Geometry check sheet. Reference: the model listing, model coordinates, mm. A direction names the side the tool comes from. Round coordinates to 2 decimals unless told otherwise and drop trailing zeros. Order: outer loops, then holes, each group sorted by start corner. A loop starts at its lowest first (then second) coordinate and runs counter-clockwise, first axis right, second up.
(1) Sectioned sample at D-D (z = 25.5). Record the boundary of the cut face in (x, y), plus the area to 3 significant figures.
(2) Set-up check for faces 4 (the face through (-11.923, 3.755, 31.944)), 5 (the face through (1.19, -5.37, 12.83)): record each of +Z, -Z, +X, -X, +Y, -Y from which the full face is reachable in a straight line by a thin tool's end or side.
(3) Sectioned sample at A-A (y = 0). Record the boundary of the cut face in (x, z), plus the area to 3 significant figures.
(4) Go/stop test with flat-tipped pins: pin 1 (8 mm diameter, centred on x = -3.5, z = 19, fed in from +Y); pin 2 (12 mm diameter, centred on x = 8, z = 13, fed in from +Y); pin 3 (5 mm diameter, centred on y = 7, z = 22, fed in from +X); pin 4 (4 mm diameter, centred on x = 0, y = 0, fed in from +Z). Record where each tip stops, or that it passes through.
(5) Sectioned sample at C-C (z = 34.5). Record the boundary of the cut face in (x, y), plus the area to 3 significant figures.
(6) Material ranges on line 1 along Y through (x, z) = (0, 13); line 2 along Z through (x, y) = (8.5, 5.5); line 3 along Z through (x, y) = (2.5, 5), recorded low to high.
(7) Release check for a two-part mould opening along Y. For faces 1 (the face through (1.73, -7.81, 25.99)), 2 (the face through (-1.7, 5.4, 25)), 3 (the face through (2.15, 0.09, 18.25)) record: +Y half, -Y half, draft (parallel to the pull), parting line (faces both ways), or undercut.
from build123d import *

# Parameters (mm, degrees)
F2_SIZE = 1
F3_R    = 1


with BuildPart() as f1:
    # F0 (on Front) → F1 (revolve)
    with BuildSketch(Plane.XZ):
        Polygon((-5.5, 0), (-2.15, 0), (-2.15, 37), (-12.5, 37), (-12.5, 27), (-8, 27), (-8, 25), (-5.5, 25), align=None)
    revolve(axis=Axis((0, 0, 18.5), (0, 0, -1)))

    # F2
    f2_edges = [f1.edges().sort_by_distance(p)[0] for p in [
        (5.5, 0, 0),
        (2.15, 0, 37),
    ]]
    chamfer(f2_edges, length=F2_SIZE)

    # F3
    f3_edges = [f1.edges().sort_by_distance(p)[0] for p in [
        (12.5, 0, 37),
        (12.5, 0, 27),
    ]]
    fillet(f3_edges, radius=F3_R)


solid = f1.part
Answer below:
1. outline: circle Ø16 at (0, 0); hole circle Ø4.3 at (0, 0)
1. area: 187 mm2
2. face 4: +Z, -Z
2. face 5: -Z
3. outline: (-12.5, 28) arc R1 ccw to (-11.5, 27) - (-8, 27) - (-8, 25) - (-5.5, 25) - (-5.5, 1) - (-4.5, 0) - (-2.15, 0) - (-2.15, 36) - (-3.15, 37) - (-11.5, 37) arc R1 ccw to (-12.5, 36) - close; (2.15, 0) - (4.5, 0) - (5.5, 1) - (5.5, 25) - (8, 25) - (8, 27) - (11.5, 27) arc R1 ccw to (12.5, 28) - (12.5, 36) arc R1 ccw to (11.5, 37) - (3.15, 37) - (2.15, 36) - close
3. area: 395 mm2
4. pin 1: stops at y = 5.5
4. pin 2: stops at y = 5.12
4. pin 3: stops at x = 3.16
4. pin 4: passes through
5. outline: circle Ø25 at (0, 0); hole circle Ø4.3 at (0, 0)
5. area: 476 mm2
6. line 1: y = -5.5 to -2.15, 2.15 to 5.5
6. line 2: z = 27 to 37
6. line 3: z = 25 to 37
7. face 1: parting line
7. face 2: draft
7. face 3: undercut
